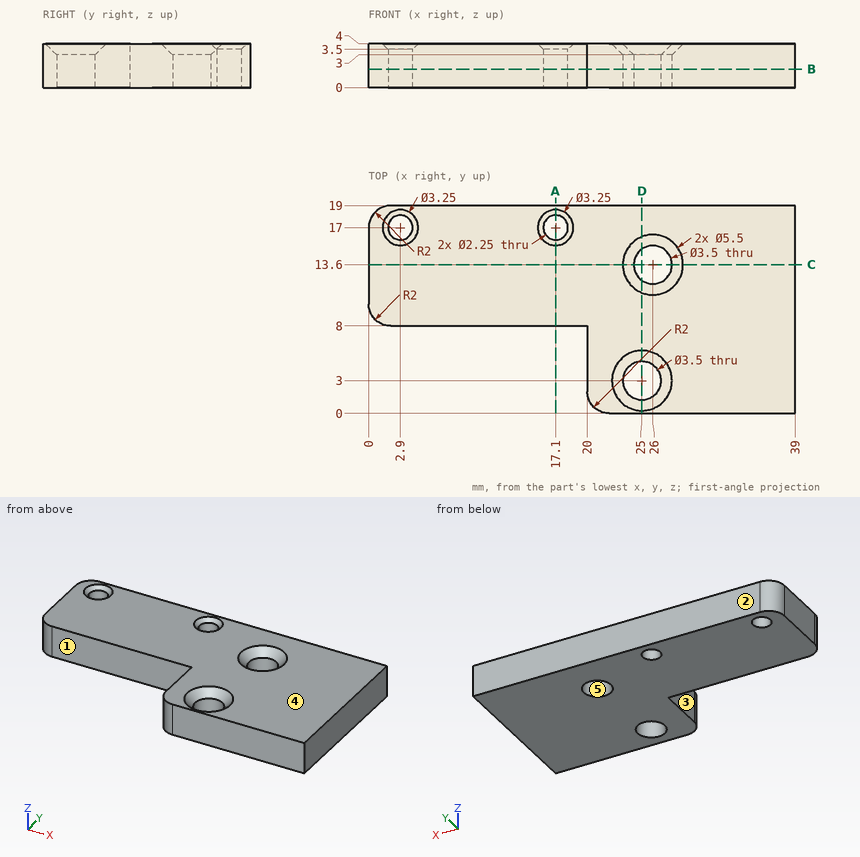
Input: dimensioned drawing with shaded views. Units: mm. Origin: part minimum x, y, z. A direction names the side the tool comes from. Give positions to 0.01 mm unless a question says otherwise; leave off trailing zeros. Write each loop counter-clockwise with the first axis right and the second up, starting at its lowest first coordinate (ties: lowest second). Pieces come first, ordered by that corner, then holes. Notation, with made-up numbers: (44.25, -13) -> (66.25, -13) arc R23 ccw to (66.25, 23) -> close; hole circle Ø9 at (-5.75, 16.5). An arc over 180 degrees is marked (long way). Return JSON: item names as keys, results as strings. Group by question number.
1. Mould query, pull axis X, two halves, no side actions, for the marked faces 3, 4 and 5. Classes: +X half, -X half, draft (parallel to the pull), parting line (faces both ways), or undercut.
2. Access query for the marked faces 1 and 2. Directions: +Z, -Z, +X, -X, +Y, -Y. A direction counts if a zero-diameter tool reaches every point of the face in a straight line with its end or side. Return the directions, or none.
3. Material intervals for line 1 (Y direction, x = 25, z = 1.2); line 2 (Y direction, x = 17.1, z = 0.7) (3 decimals); line 3 (X direction, y = 7.75, z = 2.5), sorted ascending. Write a range as from..to.
4. Pin query (flat end, axial travel): pin 1 Ø1.3 at (x, y) = (2.9, 17) entering from +Z; pin 2 Ø1.2 at (y, z) = (4, 2) entering from -X. Return the tip coordinate at first contact, or that it passes through.
5. Section D-D, the plane x = 25. Count the separate pieces of the cut face and the enclosed holes in it, then the cut area to 3 significant figures.
6. Section B-B, the plane z = 1.7. Output: boundary loops of the cut face in (x, y) (3 decimals).
7. Section A-A, the plane x = 17.1. Output: boundary loops of the cut face in (y, z) (3 decimals), then the cut area to 4 significant figures.
8. Section C-C, the plane y = 13.6. Output: boundary loops of the cut face in (x, z).
Determined:
{
 "1": {"face 3": "-X half", "face 4": "draft", "face 5": "undercut"},
 "2": {"face 1": "+Z, -Z, -X, -Y", "face 2": "+Z, -Z, +X, -X, +Y"},
 "3": {"line 1": "y = 0..1.25, 4.75..12.16, 15.04..19", "line 2": "y = 8..15.875, 18.125..19", "line 3": "x = 20..39"},
 "4": {"pin 1": "passes through", "pin 2": "stops at x = 20"},
 "5": {"separate pieces": "3", "enclosed holes": "0", "area": "48.4 mm2"},
 "6": {"outline": "(0, 10) arc R2 ccw to (2, 8) -> (20, 8) -> (20, 2) arc R2 ccw to (22, 0) -> (39, 0) -> (39, 19) -> (2, 19) arc R2 ccw to (0, 17) -> close; hole circle Ø2.25 at (2.9, 17); hole circle Ø2.25 at (17.1, 17); hole circle Ø3.5 at (25, 3); hole circle Ø3.5 at (26, 13.6)"},
 "7": {"outline": "(8, 0) -> (15.875, 0) -> (15.875, 3.5) -> (15.375, 4) -> (8, 4) -> close; (18.125, 0) -> (19, 0) -> (19, 4) -> (18.625, 4) -> (18.125, 3.5) -> close", "area": "34.75 mm2"},
 "8": {"outline": "(0, 0) -> (24.25, 0) -> (24.25, 3) -> (23.25, 4) -> (0, 4) -> close; (27.75, 0) -> (39, 0) -> (39, 4) -> (28.75, 4) -> (27.75, 3) -> close"}
}
